Model file for the job. Use its own axes, mm. Face numbers are marked on the shaded views. A direction names the side the tool comes from. Round coordinates to 2 decimals unless told otherwise and drop trailing zeros. Write each loop counter-clockwise with the first axis right and the second up, starting at its lowest first coordinate (ties: lowest second). Pieces come first, ordered by that corner, then holes. Notation, with made-up numbers: (39, 37.5) - (74, 37.5) arc R8 cw to (74, 44.5) - close; hole circle Ø5 at (-4.5, -10.75). An arc over 180 degrees is marked (long way). One line per item, written item: value.
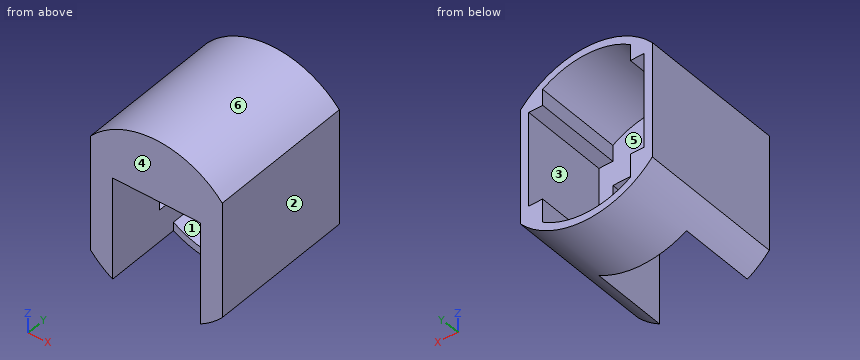
from build123d import *

# Parameters (mm, degrees)
SKETCH1_R           = 76.2
BOSS_EXTRUDE1_DEPTH = 127
CUT_EXTRUDE1_DEPTH  = 76.2
SKETCH3_W           = 76.2
SKETCH3_H           = 89.15290971
CUT_EXTRUDE2_DEPTH  = 66.04
CUT_EXTRUDE4_DEPTH  = 167.558938517
SKETCH6_W           = 100.33
SKETCH6_H           = 82.55
CUT_EXTRUDE6_DEPTH  = 76.2


with BuildPart() as part:
    # Sketch1 → Boss-Extrude1 (new body)
    with BuildSketch(Plane(origin=(0, 0, 0), x_dir=(1, 0, 0), z_dir=(0, 1, 0))):
        with Locations(Location((0, 0, 0), (0, 0, 270))):
            Circle(SKETCH1_R)
    extrude(amount=BOSS_EXTRUDE1_DEPTH)

    # Sketch2 → Cut-Extrude1 (cut)
    with BuildSketch(Plane(origin=(0, 127, 0), x_dir=(1, 0, 0), z_dir=(0, 1, 0))):
        with BuildLine():
            Line((38.1, -58.544107304), (38.1, 58.544107304))
            ThreePointArc((38.1, 58.544107304), (0, 69.85), (-38.1, 58.544107304))
            Line((-38.1, 58.544107304), (-38.1, -58.544107304))
            ThreePointArc((-38.1, -58.544107304), (0, -69.85), (38.1, -58.544107304))
        make_face()
    extrude(amount=-CUT_EXTRUDE1_DEPTH, mode=Mode.SUBTRACT)

    # Sketch3 → Cut-Extrude2 (cut)
    with BuildSketch(Plane.XZ):
        with Locations((0, -21.414680913)):
            Rectangle(SKETCH3_W, SKETCH3_H)
        with BuildLine():
            Line((38.1, -65.991135768), (-38.1, -65.991135768))
            ThreePointArc((-38.1, -65.991135768), (0, -76.2), (38.1, -65.991135768))
        make_face()
    extrude(amount=-CUT_EXTRUDE2_DEPTH, mode=Mode.SUBTRACT)

    # Sketch5 → Cut-Extrude4 (cut, through all)
    with BuildSketch(Plane(origin=(0, 127, 0), x_dir=(1, 0, 0), z_dir=(0, 1, 0))):
        with BuildLine():
            Line((-57.15, 50.401562476), (-57.15, -50.401562476))
            ThreePointArc((-57.15, -50.401562476), (-76.2, 0), (-57.15, 50.401562476))
        make_face()
        with BuildLine():
            Line((57.15, 50.401562476), (57.15, -50.401562476))
            ThreePointArc((57.15, -50.401562476), (76.2, 0), (57.15, 50.401562476))
        make_face()
    extrude(amount=-CUT_EXTRUDE4_DEPTH, mode=Mode.SUBTRACT)

    # Sketch6 → Cut-Extrude6 (cut)
    with BuildSketch(Plane(origin=(0, 127, 0), x_dir=(1, 0, 0), z_dir=(0, 1, 0))):
        with Locations((0, -3.175)):
            Rectangle(SKETCH6_W, SKETCH6_H)
    extrude(amount=-CUT_EXTRUDE6_DEPTH, mode=Mode.SUBTRACT)


solid = part.part
1. Band-saw the part on A-A on z = 9.5. Write the cut outline in (x, y) (3 decimals), plus the area to 3 significant figures.
Report:
outline: (-57.15, 0) - (-38.1, 0) - (-38.1, 50.8) - (-50.165, 50.8) - (-50.165, 127) - (-57.15, 127) - close; (38.1, 0) - (57.15, 0) - (57.15, 127) - (50.165, 127) - (50.165, 50.8) - (38.1, 50.8) - close
area: 3,000 mm²
2. Tool access for the marked faces 1, 2 and 3: list every direction of +Z, -Z, +X, -X, +Y, -Y with a clear straight run to the whole face (end or side of a thin tool).
Report:
face 1: +Y, -Y
face 2: +Z, -Z, +X, +Y, -Y
face 3: +Y
3. Band-saw the part on B-B on y = 37. Write the cut outline in (x, z), plus the area to 3 significant figures.
Report:
outline: (-57.15, -50.4) arc R76.2 ccw to (-38.1, -65.99) - (-38.1, 23.16) - (38.1, 23.16) - (38.1, -65.99) arc R76.2 ccw to (57.15, -50.4) - (57.15, 50.4) arc R76.2 ccw to (-57.15, 50.4) - close
area: 8,290 mm²
4. Wall check: probe 1 along X at (y, z) = (69, 19.5) (3 decimals); probe 2 along X at (y, z) = (25, -20.5); probe 3 along Z at (x, y) = (0.5, 43). Give the ranges that are in metal, low to high. Write a range as [from, to].
Report:
probe 1: [-57.15, -50.165], [50.165, 57.15]
probe 2: [-57.15, -38.1], [38.1, 57.15]
probe 3: [23.16, 76.2]
5. Band-saw the part on C-C on x = 19. Write the cut outline in (y, z), plus the area to 3 significant figures.
Report:
outline: (0, 23.16) - (50.8, 23.16) - (50.8, 67.22) - (127, 67.22) - (127, 73.79) - (0, 73.79) - close; (66.04, -73.79) - (127, -73.79) - (127, -67.22) - (66.04, -67.22) - close
area: 3,470 mm²
6. Band-saw the part on D-D on y = 81. Write the cut outline in (x, z) (3 decimals).
Report:
outline: (-57.15, -50.402) arc R76.2 ccw to (57.15, -50.402) - (57.15, 50.402) arc R76.2 ccw to (-57.15, 50.402) - close; hole (-50.165, -38.1) - (-38.1, -38.1) - (-38.1, -58.544) arc R69.85 ccw to (38.1, -58.544) - (38.1, -38.1) - (50.165, -38.1) - (50.165, 44.45) - (38.1, 44.45) - (38.1, 58.544) arc R69.85 ccw to (-38.1, 58.544) - (-38.1, 44.45) - (-50.165, 44.45) - close
7. Drop flat-ended pins along their axis: pin 1 (6 mm diameter, centred on x = -7.5, y = 84.5, fed in from +Z); pin 2 (5 mm diameter, centred on x = 41.5, z = 50, fed in from -Y); pin 3 (3 mm diameter, centred on x = 31.5, y = 47, fed in from +Z); pin 4 (4 mm diameter, centred on y = 103.5, z = 54.5, fed in from +X). Give the stop position or say it passes through.
Report:
pin 1: z = 76.07
pin 2: y = 0
pin 3: z = 70.05
pin 4: x = 55.23
8. Mould opens along X. For the marked faces 4, 5 and 6 say: released by +X, released by -X, zero draft, split by the parting line, or undercut.
Report:
face 4: zero draft
face 5: undercut
face 6: split by the parting line
